```python
from build123d import *

# Parameters (mm, degrees)
SKETCH2_W           = 47.65
SKETCH2_H           = 20
SKETCH2_R           = 6
BOSS_EXTRUDE1_DEPTH = 3
SKETCH3_W           = 20
SKETCH3_H           = 35
BOSS_EXTRUDE3_DEPTH = 3
SKETCH4_W           = 20
SKETCH4_H           = 35
BOSS_EXTRUDE4_DEPTH = 3
CUT_EXTRUDE1_REACH  = 67.592
SKETCH5_R           = 6
FILLET1_R           = 6.35


with BuildPart() as part:
    # Sketch2 → Boss-Extrude1 (new body)
    with BuildSketch(Plane(origin=(0, 0, 0), x_dir=(1, 0, 0), z_dir=(0, 1, 0))):
        with Locations((23.825, -10)):
            Rectangle(SKETCH2_W, SKETCH2_H)
        with Locations(Location((23.825, -10, 0), (0, 0, 270))):
            Circle(SKETCH2_R, mode=Mode.SUBTRACT)
    extrude(amount=BOSS_EXTRUDE1_DEPTH)

    # Sketch3 → Boss-Extrude3 (add)
    with BuildSketch(Plane(origin=(47.65, 0, 0), x_dir=(0, 0, -1), z_dir=(1, 0, 0))):
        with Locations((-10, -14.5)):
            Rectangle(SKETCH3_W, SKETCH3_H)
    extrude(amount=BOSS_EXTRUDE3_DEPTH)

    # Sketch4 → Boss-Extrude4 (add)
    with BuildSketch(Plane.ZY):
        with Locations((10, -14.5)):
            Rectangle(SKETCH4_W, SKETCH4_H)
    extrude(amount=BOSS_EXTRUDE4_DEPTH)

    # Cut-Extrude1: up to this face of the body (flat: up to its plane)
    cut_extrude1_end = Plane(part.part.faces().sort_by_distance((50.65, -14.5, 10))[0])
    # Sketch5 → Cut-Extrude1 (cut, up to the picked face)
    with BuildSketch(Plane.ZY.offset(3), mode=Mode.PRIVATE) as cut_extrude1_sk1:
        with Locations((10, -22)):
            Circle(SKETCH5_R)
    cut_extrude1_tool1 = split(extrude(cut_extrude1_sk1.sketch, amount=-CUT_EXTRUDE1_REACH, mode=Mode.PRIVATE), bisect_by=cut_extrude1_end, keep=Keep.BOTH, mode=Mode.PRIVATE)
    add(cut_extrude1_tool1.solids().sort_by(Axis((-3, -22, 10), (1, 0, 0)))[0], mode=Mode.SUBTRACT)

    # Fillet1
    fillet1_edges = [part.edges().sort_by_distance(p)[0] for p in [
        (49.15, -32, 20),
        (49.15, -32, 0),
        (-1.5, -32, 0),
        (-1.5, -32, 20),
    ]]
    fillet(fillet1_edges, radius=FILLET1_R)


solid = part.part
```
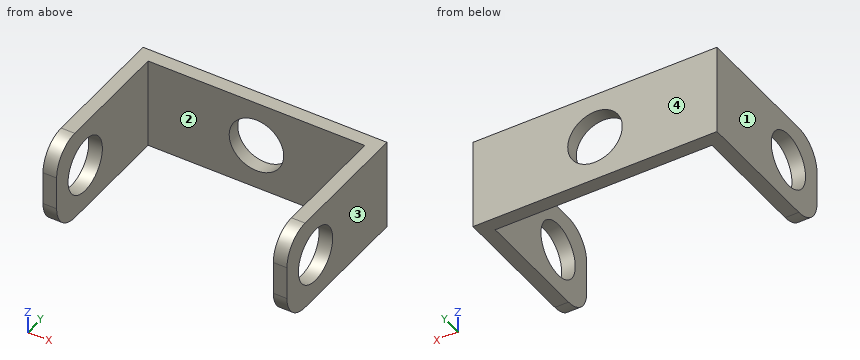
Here's how the part is built. I have some questions about the finished solid (model axes, mm). Face numbers are marked on the shaded views. Give positions to 0.01 mm unless a question says otherwise; leave off trailing zeros. Order: outer loops, then holes, each group sorted by start corner. A loop starts at its lowest first (then second) coordinate and runs counter-clockwise, first axis right, second up. Notation, with made-up numbers: (12, 1) -> (30, 1) arc R25 ccw to (30, 28) -> close; hole circle Ø2 at (7.5, 19.25). An arc over 180 degrees is marked (long way). Use CSV: the item, a comma, the result in double quotes. Start each with the question number.
Item 1: Suppose I cut it at A-A (y = -22). List the corners of the cut face in (x, z) for me, and give its area (3 significant figures).
Item 2: Thinking about a two-plate mould opening in X: for the marked faces 1, 2, 3 and 4, which applies, pulls with the +X half, pulls with the -X half, needs draft (parallel to the pull), parting line crosses it, or undercut?
Item 3: Suppose I cut it at D-D (x = 27). List the corners of the cut face in (y, z) for me, and give its area (3 significant figures).
Item 4: I'm going to push flat-ended pins straight in: P1, Ø6, axis at x = 27, z = 11.5, coming from the -Y side; P2, Ø6, axis at y = -21, z = 10, coming from the -X side. Where does each tip first touch, or does it pass through?
Item 5: Suppose I cut it at B-B (z = 10). List the corners of the cut face in (x, y) for me (3 decimals).
Item 6: If I drill on probe 1 along Y at (x, z) = (-2.2, 10); probe 2 along X at (y, z) = (-29.5, 12.5); probe 3 along X at (y, z) = (2.1, 10) (3 decimals), over which ranges is the centre line in solid material (lowest first)? Write a range as [from, to].
Item 7: Suppose I cut it at C-C (y = -4). List the corners of the cut face in (x, z) for me.
Answer block:
1,outline,"(-3, 0) -> (0, 0) -> (0, 4) -> (-3, 4) -> close; (-3, 16) -> (0, 16) -> (0, 20) -> (-3, 20) -> close; (47.65, 0) -> (50.65, 0) -> (50.65, 4) -> (47.65, 4) -> close; (47.65, 16) -> (50.65, 16) -> (50.65, 20) -> (47.65, 20) -> close"
1,area,"48.0 mm^2"
2,face 1,"pulls with the -X half"
2,face 2,"undercut"
2,face 3,"pulls with the +X half"
2,face 4,"needs draft"
3,outline,"(0, 0) -> (3, 0) -> (3, 4.91) -> (0, 4.91) -> close; (0, 15.09) -> (3, 15.09) -> (3, 20) -> (0, 20) -> close"
3,area,"29.5 mm^2"
4,P1,"stops at y = 0"
4,P2,"passes through"
5,outline,"(-3, -32) -> (0, -32) -> (0, -28) -> (-3, -28) -> close; (-3, -16) -> (0, -16) -> (0, 0) -> (17.825, 0) -> (17.825, 3) -> (-3, 3) -> close; (29.825, 0) -> (47.65, 0) -> (47.65, -16) -> (50.65, -16) -> (50.65, 3) -> (29.825, 3) -> close; (47.65, -32) -> (50.65, -32) -> (50.65, -28) -> (47.65, -28) -> close"
6,probe 1,"y = [-32, -28], [-16, 3]"
6,probe 2,"x = [-3, 0], [47.65, 50.65]"
6,probe 3,"x = [-3, 17.825], [29.825, 50.65]"
7,outline,"(-3, 0) -> (0, 0) -> (0, 20) -> (-3, 20) -> close; (47.65, 0) -> (50.65, 0) -> (50.65, 20) -> (47.65, 20) -> close"
